Source: CAD feature listing. Evaluate the final solid. Frame: model axes, mm. A direction names the side the tool comes from. Coordinates: 2 decimals unless noted, no trailing zeros. Write each loop counter-clockwise with the first axis right and the second up, starting at its lowest first coordinate (ties: lowest second). Pieces come first, ordered by that corner, then holes. Notation, with made-up numbers: M -30.5,85 L 25.5,85 A31 cw 25.5,111 Z; hole C 75,15.5 d3. An arc over 180 degrees is marked long. Write item = value, one per line. Start each with the question number.
1. Section query D-D (y = -6.35). Give the number of separate pieces and of enclosed holes in the cut face, then the cut area to 3 significant figures.
2. Access query for faces 1 (the face through (50.13, -6.01, 53.25)), 2 (the face through (80, -3, 59)). Directions: +Z, -Z, +X, -X, +Y, -Y. A direction counts if a zero-diameter tool reaches every point of the face in a straight line with its end or side. Return the directions, or none.
3. Section query B-B (z = 55.5). Output: boundary loops of the cut face in (x, y), then the cut area to 3 significant figures.
4. Pull-direction query (X, two-part tool) for faces 3 (the face through (79, -7, 32)), 4 (the face through (79, -5, 31)); classes: pulls with the +X half, pulls with the -X half, needs draft (parallel to the pull), parting line crosses it, or undercut.
5. Section query C-C (x = 39). Output: boundary loops of the cut face in (y, z), then the cut area to 3 significant figures.
6. Pin query (flat end, axial travel): pin 1 Ø4 at (x, z) = (144, 45) entering from +Y; pin 2 Ø0.5 at (x, y) = (164, -4) entering from -Z; pin 3 Ø0.6 at (y, z) = (-3.5, 61.5) entering from -X. Return the tip coordinate at first contact, or that it passes through.
7. Section query A-A (x = 8.5). Output: boundary loops of the cut face in (y, z).
8. Line query: line 1 along Z through (x, y) = (162.5, -5.6); line 2 along X through (y, z) = (-5.45, 60.5); line 3 along X through (y, z) = (-6.75, 20). Output: solid intervals per line, ascending.
```python
from build123d import *

# Parameters (mm, degrees)
PAD004_DEPTH    = 2
SKETCH008_W     = 169
SKETCH008_H     = 61.7
PAD005_DEPTH    = 2
SKETCH009_R     = 2.2
POCKET002_DEPTH = 4.001
SKETCH012_W     = 159
SKETCH012_H     = 51.7
POCKET005_DEPTH = 2
SKETCH010_R     = 4.5
SKETCH010_W     = 13
SKETCH010_H     = 19
POCKET003_DEPTH = 4.001


with BuildPart() as part:
    # Sketch007 → Pad004 (new body)
    with BuildSketch(Plane.XZ):
        with BuildLine():
            Line((-2, 62.7), (-2, 0))
            ThreePointArc((-2, 0), (-1.414214, -1.414214), (0, -2))
            Line((0, -2), (170, -2))
            ThreePointArc((170, -2), (171.414214, -1.414214), (172, 0))
            Line((172, 0), (172, 62.7))
            ThreePointArc((172, 62.7), (171.414214, 64.114214), (170, 64.7))
            Line((170, 64.7), (0, 64.7))
            ThreePointArc((0, 64.7), (-1.414214, 64.114214), (-2, 62.7))
        make_face()
    extrude(amount=PAD004_DEPTH)

    # Sketch008 (on Face9 of Pad004) → Pad005 (join)
    with BuildSketch(Plane(origin=(0, 0, 0), x_dir=(1, 0, 0), z_dir=(0, 1, 0))):
        with Locations((85, -31.35)):
            Rectangle(SKETCH008_W, SKETCH008_H)
    extrude(amount=PAD005_DEPTH)

    # Sketch009 (on Face5 of Pad005) → Pocket002 (cut, through all)
    with BuildSketch(Plane.XZ.offset(2)):
        with Locations((2.5, 2.5)):
            Circle(SKETCH009_R)
        with Locations((2.5, 60.5)):
            Circle(SKETCH009_R)
        with Locations((167.5, 60.5)):
            Circle(SKETCH009_R)
        with Locations((167.5, 2.5)):
            Circle(SKETCH009_R)
    extrude(amount=-POCKET002_DEPTH, mode=Mode.SUBTRACT)

    # Sketch012 (on Face28 of Pocket002) → Pocket005 (cut)
    with BuildSketch(Plane(origin=(0, 2, 0), x_dir=(1, 0, 0), z_dir=(0, 1, 0))):
        with Locations((85, -31.35)):
            Rectangle(SKETCH012_W, SKETCH012_H)
    extrude(amount=-POCKET005_DEPTH, mode=Mode.SUBTRACT)


with BuildPart() as part_1:
    # Body003 placement: moved
    add(part.part.moved(Location((-5, -5, 0))))


with BuildPart() as part_2:
    # BaseFeature placement: moved
    add(part_1.part.moved(Location((5, 5, 0))))

    # Sketch010 (on Face5 of BaseFeature) → Pocket003 (cut, through all)
    with BuildSketch(Plane.XZ.offset(2)):
        with Locations((12, 45)):
            Circle(SKETCH010_R)
        with Locations((28.5, 44.5)):
            Rectangle(SKETCH010_W, SKETCH010_H)
        with BuildLine():
            Line((62.5, 23.436932), (62.5, 16.563068))
            ThreePointArc((47.5, 16.563068), (55, 11.75), (62.5, 16.563068))
            Line((47.5, 23.436932), (47.5, 16.563068))
            ThreePointArc((62.5, 23.436932), (55, 28.25), (47.5, 23.436932))
        make_face()
        with BuildLine():
            ThreePointArc((47.5, 41.563068), (55, 36.75), (62.5, 41.563068))
            Line((62.5, 48.436932), (62.5, 41.563068))
            ThreePointArc((62.5, 48.436932), (55, 53.25), (47.5, 48.436932))
            Line((47.5, 48.436932), (47.5, 41.563068))
        make_face()
        with BuildLine():
            ThreePointArc((87.5, 23.436932), (80, 28.25), (72.5, 23.436932))
            Line((72.5, 23.436932), (72.5, 16.563068))
            ThreePointArc((72.5, 16.563068), (80, 11.75), (87.5, 16.563068))
            Line((87.5, 23.436932), (87.5, 16.563068))
        make_face()
        with BuildLine():
            Line((97.5, 23.436932), (97.5, 16.563068))
            ThreePointArc((97.5, 16.563068), (105, 11.75), (112.5, 16.563068))
            Line((112.5, 23.436932), (112.5, 16.563068))
            ThreePointArc((112.5, 23.436932), (105, 28.25), (97.5, 23.436932))
        make_face()
        with BuildLine():
            Line((72.5, 48.436932), (72.5, 41.563068))
            ThreePointArc((72.5, 41.563068), (80, 36.75), (87.5, 41.563068))
            Line((87.5, 48.436932), (87.5, 41.563068))
            ThreePointArc((87.5, 48.436932), (80, 53.25), (72.5, 48.436932))
        make_face()
    extrude(amount=-POCKET003_DEPTH, mode=Mode.SUBTRACT)


with BuildPart() as part_3:
    # Body004 placement: moved
    add(part_2.part.moved(Location((-5, -5, 0))))


solid = part_3.part
```
Results are:
q1.separate_pieces = 1
q1.enclosed_holes = 11
q1.area = 10,200 mm^2
q2.face_1 = +Y, -Y
q2.face_2 = +Z, -Z, +X, -X, +Y
q3.outline = M -7,-7 L 167,-7 L 167,-5 L 164.5,-5 L 164.5,-3 L 159.5,-3 L 159.5,-5 L 0.5,-5 L 0.5,-3 L -4.5,-3 L -4.5,-5 L -7,-5 Z
q3.area = 368 mm^2
q4.face_3 = needs draft
q4.face_4 = undercut
q5.outline = M -7,-2 L -5,-2 L -5,0.5 L -3,0.5 L -3,5.5 L -5,5.5 L -5,57.2 L -3,57.2 L -3,62.2 L -5,62.2 L -5,64.7 L -7,64.7 Z
q5.area = 153 mm^2
q6.pin_1 = -5
q6.pin_2 = 0.5
q6.pin_3 = -4.5
q7.outline = M -7,-2 L -5,-2 L -5,0.5 L -3,0.5 L -3,5.5 L -5,5.5 L -5,40.76 L -7,40.76 Z; M -7,49.24 L -5,49.24 L -5,57.2 L -3,57.2 L -3,62.2 L -5,62.2 L -5,64.7 L -7,64.7 Z
q8.line_1 = -2 to 0.3, 4.7 to 58.3, 62.7 to 64.7
q8.line_2 = -7 to -4.7, -0.3 to 160.3, 164.7 to 167
q8.line_3 = -7 to 42.5, 57.5 to 67.5, 82.5 to 92.5, 107.5 to 167
